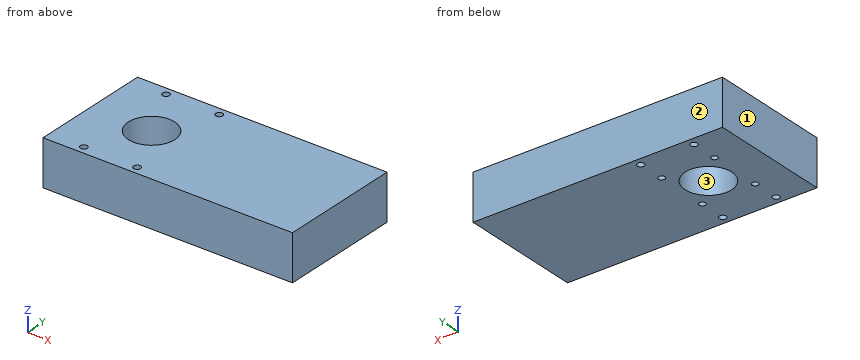
from build123d import *

# Parameters (mm, degrees)
F0_W     = 118
F0_H     = 58
F0_R     = 1.65
F0_R_2   = 11
F1_DEPTH = 21.6
F2_D     = 3
F2_DEPTH = 5
F2_TIP   = 0.9012909285


with BuildPart() as f1:
    # F0 (on Top) → F1 (new body)
    with BuildSketch(Plane.XY):
        with Locations((4.9529026613, -7.0896845311)):
            Rectangle(F0_W, F0_H)
        with Locations((-37.6470973387, -32.2896845311)):
            Circle(F0_R, mode=Mode.SUBTRACT)
        with Locations((-12.4470973387, -32.2896845311)):
            Circle(F0_R, mode=Mode.SUBTRACT)
        with Locations((-25.0470973387, -7.0896845311)):
            Circle(F0_R_2, mode=Mode.SUBTRACT)
        with Locations((-37.6470973387, 18.1103154689)):
            Circle(F0_R, mode=Mode.SUBTRACT)
        with Locations((-12.4470973387, 18.1103154689)):
            Circle(F0_R, mode=Mode.SUBTRACT)
    extrude(amount=F1_DEPTH)

    # F2
    with Locations(Plane(origin=(0, 0, 0), x_dir=(1, 0, 0), z_dir=(0, 0, -1))):
        with Locations((-37.5470973387, 19.5896845311), (-12.5470973387, 19.5896845311), (-12.5470973387, -5.4103154689), (-37.5470973387, -5.4103154689)):
            Hole(F2_D / 2, depth=F2_DEPTH)
            with Locations((0, 0, -(F2_DEPTH + F2_TIP / 2))):  # 118° drill point
                Cone(0, F2_D / 2, F2_TIP, mode=Mode.SUBTRACT)


solid = f1.part
The listing builds one solid part. Answer for the finished solid, in the listing's coordinates (mm). Face numbers are marked on the shaded views. Give positions to 0.01 mm unless a question says otherwise; leave off trailing zeros. Write each loop counter-clockwise with the first axis right and the second up, starting at its lowest first coordinate (ties: lowest second). Pieces come first, ordered by that corner, then holes.
Item 1: Find the intervals of material crossed by line 1 along X through (y, z) = (-7.5, 17.5); line 2 along X through (y, z) = (19, 5); line 3 along X through (y, z) = (1, 12.75), in increasing order.
Item 2: Flat-ended cylindrical pins translate along their axes: P1, Ø20, axis at x = -25.05, y = -7.09, coming from the -Z side; P2, Ø2.5, axis at x = -12.55, y = -19.59, coming from the -Z side; P3, Ø1.8, axis at x = -37.55, y = 5.41, coming from the -Z side. Find the tip coordinate at first contact, or state that the pin passes through.
Item 3: Determine the mould class of the marked faces 1, 2 and 3 for opening direction Y: released by +Y, released by -Y, zero draft, split by the parting line, or undercut.
Item 4: Section A-A, the plane y = 1 is taken. Write down the section's boundary in (x, z).
Item 5: Section C-C, the plane z = 13.5 is taken. Write down the section's boundary in (x, y), plus the area to 3 significant figures.
Item 6: Section D-D, the plane z = 3.75 is taken. Count the separate pieces of the cut face and the enclosed holes in it, plus the area to 3 significant figures.
Item 7: Section B-B, the plane x = -18.5 is taken. Write down the section's boundary in (y, z), plus the area to 3 significant figures.
Completed:
1. line 1: x = -54.05 to -36.04, -14.05 to 63.95
1. line 2: x = -54.05 to -39.04, -36.26 to -13.84, -11.06 to 63.95
1. line 3: x = -54.05 to -32.5, -17.59 to 63.95
2. P1: passes through
2. P2: stops at z = 5.15
2. P3: stops at z = 5.36
3. face 1: zero draft
3. face 2: released by +Y
3. face 3: undercut
4. outline: (-54.05, 0) - (-32.5, 0) - (-32.5, 21.6) - (-54.05, 21.6) - close; (-17.59, 0) - (63.95, 0) - (63.95, 21.6) - (-17.59, 21.6) - close
5. outline: (-54.05, -36.09) - (63.95, -36.09) - (63.95, 21.91) - (-54.05, 21.91) - close; hole circle Ø3.3 at (-37.65, -32.29); hole circle Ø3.3 at (-37.65, 18.11); hole circle Ø22 at (-25.05, -7.09); hole circle Ø3.3 at (-12.45, -32.29); hole circle Ø3.3 at (-12.45, 18.11)
5. area: 6,430 mm2
6. separate pieces: 1
6. enclosed holes: 9
6. area: 6,400 mm2
7. outline: (-36.09, 0) - (-15.93, 0) - (-15.93, 21.6) - (-36.09, 21.6) - close; (1.75, 0) - (21.91, 0) - (21.91, 21.6) - (1.75, 21.6) - close
7. area: 871 mm2
